Model file for the job. Use its own axes, mm. A direction names the side the tool comes from. Coordinates: 2 decimals unless noted, no trailing zeros. Loops run counter-clockwise (first coordinate to the right, second up) from the corner with the lowest first, then second, coordinate; pieces in that order, holes last.
Solid Edge part; units mm, degrees
sketch "Sketch1" plane through (0, 0, 0) normal (0, -1, 0) x (1, 0, 0)
  line L0 (10, 4) -> (10, 0)
  line L1 (10, 0) -> (8.6, 0)
  line L2 (8.6, 0) -> (8.6, 4)
  line L3 (8.6, 4) -> (7.8, 4)
  line L4 (7.8, 4) -> (7.8, 10)
  line L5 (7.8, 10) -> (9, 10)
  line L6 (9, 10) -> (9, 4)
  line L7 (9, 4) -> (10, 4)
revolve "RevolvedProtrusion1" add sketch "Sketch1" angle 360 about axis through (0, 0, 0) along (0, 0, 1)
sketch "Sketch2" plane through (0, 0, 10) normal (0, 0, 1) x (1, 0, 0)
  line L0 (-13.844, -3.125) -> (13.844, -3.125)
  line L1 (13.844, -3.125) -> (13.844, 3.125)
  line L2 (13.844, 3.125) -> (-13.844, 3.125)
  line L3 (-13.844, 3.125) -> (-13.844, -3.125)
extrude "Cutout1" cut sketch "Sketch2" against normal up to surface (6 mm away)
fillet "Round1" radius 0.4 4 edges at (0, 8.6, 4) (0, -8.6, 4) (0, -7.8, 4) (0, 7.8, 4)
chamfer "Chaflán_1" distance 0.2 angle 45 1 edges at (-8.6, 0, 0)
Q1. Flat gauge pins, fed straight in: P1, Ø10, axis at x = -3.5, y = 1.5, coming from the +Z side; P2, Ø1, axis at x = 7.5, z = 5.5, coming from the +Y side; P3, Ø1, axis at x = 2.5, z = 1.5, coming from the -Y side; P4, Ø6, axis at y = -4.5, z = 1.5, coming from the -X side. Where does each tip first touch, or does it go through?
Answers:
P1: stops at z = 10
P2: stops at y = 5.66
P3: stops at y = -9.8
P4: stops at x = -9.89
Q2. Which spindle directions (+Z, -Z, +X, -X, +Y, -Y) get a long thin tool onto all of the face, cutting with end or side? Do faces 4 (the cylindrical face through (0, -9, 7)), 5 (the cylindrical face through (-0.1, -7.8, 7.2)), 6 (the flat face through (-9, -1, 4)), 7 (the flat face through (-1, -8, 10)), 8 (the cylindrical face through (-1.12, 8.527, 2.127)). Say none if no direction does.
Answers:
face 4: +Z, -Y
face 5: +Z, -Z
face 6: +Z
face 7: +Z, +X, -X, +Y, -Y
face 8: -Z
Q3. Mould opens along X. For faces 1 (the cylindrical face through (0, 9, 7)), 2 (the flat face through (0, 8, 10)), 3 (the cylindrical face through (0.1, 7.8, 7.2)) say: +X half, -X half, draft (parallel to the pull), parting line (faces both ways), or undercut.
Answers:
face 1: parting line
face 2: draft
face 3: undercut
Q4. Drill centre lines: line 1 (Y direction, x = 0, z = 1.35); line 2 (X direction, y = -7.75, z = 2.5). Where is each one in solid material? Low to high.
Answers:
line 1: y = -10 to -8.6, 8.6 to 10
line 2: x = -6.32 to -3.73, 3.73 to 6.32
Q5. Slice it at C-C (x = 0). List the corners of the cut face in (y, z), and give its area (3 significant figures).
Answers:
outline: (-10, 0) - (-8.8, 0) - (-8.6, 0.2) - (-8.6, 3.6) arc R0.4 cw to (-8.2, 4) arc R0.4 ccw to (-7.8, 4.4) - (-7.8, 10) - (-9, 10) - (-9, 4) - (-10, 4) - close; (7.8, 4.4) arc R0.4 ccw to (8.2, 4) arc R0.4 cw to (8.6, 3.6) - (8.6, 0.2) - (8.8, 0) - (10, 0) - (10, 4) - (9, 4) - (9, 10) - (7.8, 10) - close
area: 25.6 mm2
Q6. Slice it at B-B (z = 7). List the corners of the cut face in (x, y) (3 decimals).
Answers:
outline: (-8.44, -3.125) arc R9 ccw to (8.44, -3.125) - (7.147, -3.125) arc R7.8 cw to (-7.147, -3.125) - close; (-8.44, 3.125) - (-7.147, 3.125) arc R7.8 cw to (7.147, 3.125) - (8.44, 3.125) arc R9 ccw to start
Q7. Slice it at D-D (z = 2). List the corners of the cut face in (x, y).
Answers:
outline: circle Ø20 at (0, 0); hole circle Ø17.2 at (0, 0)
Q8. Slice it at A-A (y = 0). List the corners of the cut face in (x, z), and give its area (3 significant figures).
Answers:
outline: (-10, 0) - (-8.8, 0) - (-8.6, 0.2) - (-8.6, 4) - (-10, 4) - close; (8.6, 0.2) - (8.8, 0) - (10, 0) - (10, 4) - (8.6, 4) - close
area: 11.2 mm2
